Check sheet for the drawn part. Datum: minimum x, y, z corner. Units: mm. A direction names the side the tool comes from. Round coordinates to 2 decimals unless told otherwise and drop trailing zeros. Order: outer loops, then holes, each group sorted by start corner. A loop starts at its lowest first (then second) coordinate and runs counter-clockwise, first axis right, second up. Notation, with made-up numbers: (10, 6.5) -> (36, 6.5) arc R21 cw to (36, 15.5) -> close; hole circle Ø5 at (45.25, 17). An arc over 180 degrees is marked (long way). Answer as a JSON object with one key per item and string values. Group by question number.
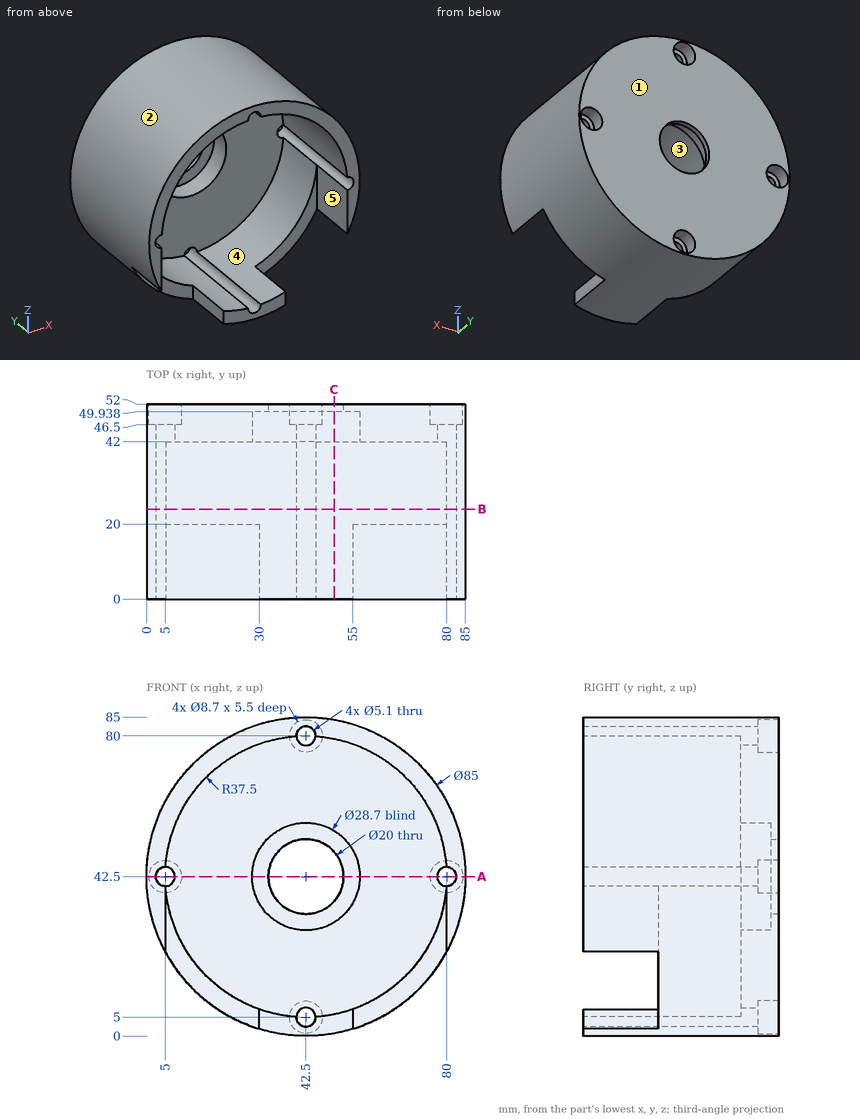
Item 1: Depth check by flat-ended pin: pin 1 Ø5 at (x, z) = (5, 42.5) entering from -Y; pin 2 Ø4 at (y, z) = (27, 15.5) entering from -X; pin 3 Ø4.5 at (x, z) = (5, 44) entering from +Y; pin 4 Ø3 at (y, z) = (26.5, 11) entering from +X (1 decimal). Enter the tip coordinate at first touch or a pass-through.
Item 2: Sectioned sample at B-B, the plane y = 24. Enter the section's corners in (x, z).
Item 3: Mould release check, pull along X, two halves, no side actions. Record for the marked faces 1, 2 and 3: pulls with the +X half, pulls with the -X half, needs draft (parallel to the pull), parting line crosses it, or undercut.
Item 4: Thickness scan on L1, parallel to Z at x = 42.5, y = 20.5; L2, parallel to X at y = 48, z = 42.5; L3, parallel to X at y = 50, z = 42. Record the ranges inside material, lowest first.
Item 5: Set-up check for the marked faces 4 and 5: record each of +Z, -Z, +X, -X, +Y, -Y from which the full face is reachable in a straight line by a thin tool's end or side.
Item 6: Sectioned sample at C-C, the plane x = 50. Enter the section's corners in (y, z) (1 decimal), then the cut area to 3 significant figures.
Item 7: Sectioned sample at A-A, the plane z = 42.5. Enter the section's corners in (x, y).
Result:
{
 "1": {"pin 1": "passes through", "pin 2": "stops at x = 8.13", "pin 3": "stops at y = 46.5", "pin 4": "stops at x = 72.6"},
 "2": {"outline": "circle Ø85 at (42.5, 42.5); hole (5.09, 39.95) arc R37.5 ccw to (39.95, 5.09) arc R2.55 ccw (long way) to (45.05, 5.09) arc R37.5 ccw to (79.91, 39.95) arc R2.55 ccw (long way) to (79.91, 45.05) arc R37.5 ccw to (45.05, 79.91) arc R2.55 ccw (long way) to (39.95, 79.91) arc R37.5 ccw to (5.09, 45.05) arc R2.55 ccw (long way) to start"},
 "3": {"face 1": "needs draft", "face 2": "parting line crosses it", "face 3": "undercut"},
 "4": {"L1": "z = 0 to 2.45, 82.55 to 85", "L2": "x = 0 to 0.65, 9.35 to 28.15, 56.85 to 75.65, 84.35 to 85", "L3": "x = 0 to 0.68, 9.32 to 32.51, 52.49 to 75.68, 84.32 to 85"},
 "5": {"face 4": "-Y", "face 5": "-Z, -Y"},
 "6": {"outline": "(0, 0.7) -> (52, 0.7) -> (52, 35.9) -> (49.9, 35.9) -> (49.9, 30.3) -> (42, 30.3) -> (42, 5.8) -> (0, 5.8) -> close; (0, 79.2) -> (42, 79.2) -> (42, 54.7) -> (49.9, 54.7) -> (49.9, 49.1) -> (52, 49.1) -> (52, 84.3) -> (0, 84.3) -> close", "area": "1,040 mm2"},
 "7": {"outline": "(0, 0) -> (2.45, 0) -> (2.45, 46.5) -> (0.65, 46.5) -> (0.65, 52) -> (0, 52) -> close; (7.55, 42) -> (28.15, 42) -> (28.15, 49.94) -> (32.5, 49.94) -> (32.5, 52) -> (9.35, 52) -> (9.35, 46.5) -> (7.55, 46.5) -> close; (52.5, 49.94) -> (56.85, 49.94) -> (56.85, 42) -> (77.45, 42) -> (77.45, 46.5) -> (75.65, 46.5) -> (75.65, 52) -> (52.5, 52) -> close; (82.55, 0) -> (85, 0) -> (85, 52) -> (84.35, 52) -> (84.35, 46.5) -> (82.55, 46.5) -> close"}
}
